Source: CAD feature listing. Evaluate the final solid. Frame: model axes, mm. Face numbers are marked on the shaded views. A direction names the side the tool comes from. Round coordinates to 2 decimals unless told otherwise and drop trailing zeros. Order: outer loops, then holes, each group sorted by start corner. A loop starts at its lowest first (then second) coordinate and runs counter-clockwise, first axis right, second up. Notation, with made-up numbers: (41.5, 43) -> (91.5, 43) arc R17 cw to (91.5, 76) -> close; hole circle Ø2 at (-18.75, 86.25). An arc over 180 degrees is marked (long way). Write item = value, one per line. Start each with the question number.
(1) Contact query for flat-ended pins moving along their axis: pin 1 Ø1.5 at (x, y) = (10, 0) entering from +Z; pin 2 Ø1 at (y, z) = (-1, -5.5) entering from +X; pin 3 Ø3 at (y, z) = (2.5, 4) entering from +X. Output: stop coordinate, or through.
(2) Cut plane D-D on z = 3.75. Return the cut outline in (x, y).
(3) Reachability of the marked faces 4, 5 and 6 from +Z, -Z, +X, -X, +Y, -Y: full face, straight path, thin tool, end or side. Return the list, or none.
(4) Cut plane A-A on y = 0.5. Return the cut outline in (x, z), then the cut area to 3 significant figures.
(5) Cut plane B-B on z = 0. Return the cut outline in (x, y).
(6) Ray query, line 1 (X direction, y = 0.2, z = -0.5); line 2 (Y direction, x = 12.6, z = 0.45); line 3 (Z direction, x = 0, y = -0.75). Return the intervals inside material, ascending.
(7) Draft query along X for the marked faces 1, 2 and 3. Return one class per face: released by +X, released by -X, zero draft, split by the parting line, or undercut.
(8) Cut plane C-C on x = 0. Return the cut outline in (y, z).
Autodesk Inventor part; units mm, degrees
ref_plane "YZ Plane" through (0, 0, 0) normal (1, 0, 0) x (0, 1, 0)
ref_plane "XZ Plane" through (0, 0, 0) normal (0, 1, 0) x (-1, 0, 0)
ref_plane "XY Plane" through (0, 0, 0) normal (0, 0, 1) x (1, 0, 0)
sketch "Sketch1" plane through (0, 0, 0) normal (0, 1, 0) x (-1, 0, 0)
  circle A0 centre (0, 0) radius 4
  circle A1 centre (0, 0) radius 5.6
  circle A2 centre (0, 0) radius 7.6
  dimension "d0" = 8
  dimension "d1" = 11.2
  dimension "d14" = 2
extrude "Extrusion1" add sketch "Sketch1" against normal blind 2 contours A1 | A2
extrude "Extrusion2" add sketch "Sketch1" along normal blind 3 contours A2
sketch "Sketch2" plane through (0, 0, 0) normal (0, 0, 1) x (1, 0, 0)
  line L0 (7.6, 3) -> (7.6, -2)
  line L1 (7.6, 3) -> (12.6, 3)
  line L2 (7.6, -2) -> (12.6, -2)
  line L3 (7.6, 0.5) -> (12.6, 0.5) construction
  circle A0 centre (12.6, 0.5) radius 2.5
  circle A1 centre (12.6, 0.5) radius 1.1
  line L4 (7.6, 3) -> (6.6, 3)
  line L5 (6.6, 3) -> (6.6, -2)
  line L6 (6.6, -2) -> (7.6, -2)
  point P0 (0, 0)
  dimension "d7" = 2.2
  dimension "d8" = 5
  dimension "d11" = 1
  dimension "d15" = 5
extrude "Extrusion3" add sketch "Sketch2" along normal mid plane 2
properties part number "Bearing Grip_3DPrint"
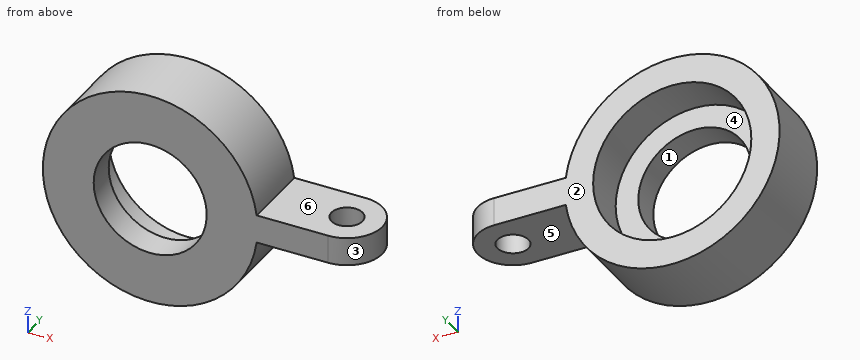
Evaluation:
q1.pin_1 = 1
q1.pin_2 = 5.72
q1.pin_3 = 7.18
q2.outline = (-6.61, -2) -> (-1.39, -2) -> (-1.39, 0) -> (-4.16, 0) -> (-4.16, 3) -> (-6.61, 3) -> close; (1.39, -2) -> (6.61, -2) -> (6.61, 3) -> (4.16, 3) -> (4.16, 0) -> (1.39, 0) -> close
q3.face_4 = +Y
q3.face_5 = -Z, +X, +Y, -Y
q3.face_6 = +Z, +X, +Y, -Y
q4.outline = (7.53, -1) -> (11.5, -1) -> (11.5, 1) -> (7.53, 1) arc R7.6 ccw (long way) to start; (13.7, -1) -> (15.1, -1) -> (15.1, 1) -> (13.7, 1) -> close; hole circle Ø11.2 at (0, 0)
q4.area = 93.6 mm^2
q5.outline = (-7.6, -2) -> (-4, -2) -> (-4, 0) -> (-5.6, 0) -> (-5.6, 3) -> (-7.6, 3) -> close; (4, -2) -> (12.6, -2) arc R2.5 ccw to (12.6, 3) -> (5.6, 3) -> (5.6, 0) -> (4, 0) -> close; hole circle Ø2.2 at (12.6, 0.5)
q6.line_1 = -7.58 to -5.58, 5.58 to 11.54, 13.66 to 15.08
q6.line_2 = -2 to -0.6, 1.6 to 3
q6.line_3 = -7.6 to -4, 4 to 7.6
q7.face_1 = undercut
q7.face_2 = zero draft
q7.face_3 = released by +X
q8.outline = (-2, -7.6) -> (3, -7.6) -> (3, -5.6) -> (0, -5.6) -> (0, -4) -> (-2, -4) -> close; (-2, 4) -> (0, 4) -> (0, 5.6) -> (3, 5.6) -> (3, 7.6) -> (-2, 7.6) -> close
